from build123d import *

# Parameters (mm, degrees)
SKETCH_1_W          = 30.50790567
SKETCH_1_H          = 76
SKETCH_1_R          = 1.716069694
SKETCH_1_W_2        = 11.5
SKETCH_1_H_2        = 11.5
SKETCH_1_W_3        = 24.50790567
SKETCH_1_H_3        = 19
EXTRUDE_1_DEPTH     = 3.3
SKETCH_2_W          = 30.50790567
SKETCH_2_H          = 6
EXTRUDE_2_DEPTH     = 1
EXTRUDE_3_DEPTH     = 3.3
CUT_EXTRUDE_1_DEPTH = 3.3
SKETCH_8_W          = 30.50790567
SKETCH_8_H          = 29
EXTRUDE_5_DEPTH     = 3.3
CUT_EXTRUDE_3_DEPTH = 3.3
SKETCH_12_W         = 4.466233575
SKETCH_12_H         = 76.29690536
SKETCH_12_W_2       = 3.912291759
SKETCH_12_H_2       = 55.852177881
CUT_EXTRUDE_6_DEPTH = 11.3


with BuildPart() as part:
    # 草圖1 → 填料-伸長1 (new body)
    with BuildSketch(Plane.XY):
        with Locations((0, -4.833822083)):
            Rectangle(SKETCH_1_W, SKETCH_1_H)
        with Locations((-8.65, 10.166177917)):
            Circle(SKETCH_1_R, mode=Mode.SUBTRACT)
        with Locations((-0.03771926, 22.181861337)):
            Rectangle(SKETCH_1_W_2, SKETCH_1_H_2, mode=Mode.SUBTRACT)
        with Locations((8.65, 10.166177917)):
            Circle(SKETCH_1_R, mode=Mode.SUBTRACT)
        with Locations((0, -30.333822083)):
            Rectangle(SKETCH_1_W_3, SKETCH_1_H_3, mode=Mode.SUBTRACT)
    extrude(amount=EXTRUDE_1_DEPTH)

    # 草圖2 → 填料-伸長2 (add)
    with BuildSketch(Plane.XY.offset(3.3)):
        with Locations((0, 1.166177917)):
            Rectangle(SKETCH_2_W, SKETCH_2_H)
        with Locations((0, -10.833822083)):
            Rectangle(SKETCH_2_W, SKETCH_2_H)
    extrude(amount=EXTRUDE_2_DEPTH)

    # 草圖3 → 填料-伸長3 (add)
    with BuildSketch(Plane.XY):
        Polygon((15.253952835, -42.833822083), (-15.253952835, -18.474060109), (15.253952835, -18.474060109), align=None)
    extrude(amount=EXTRUDE_3_DEPTH)

    # 草圖4 → 除料-伸長1 (cut)
    with BuildSketch(Plane.XY.offset(3.3)):
        Polygon((15.253952835, -42.833822083), (-15.253952835, -18.806748841), (-15.253952835, -42.833822083), align=None)
    extrude(amount=-CUT_EXTRUDE_1_DEPTH, mode=Mode.SUBTRACT)

    # 草圖8 → 填料-伸長5 (add)
    with BuildSketch(Plane.XY.offset(3.3)):
        with Locations((0, -28.333822083)):
            Rectangle(SKETCH_8_W, SKETCH_8_H)
    extrude(amount=-EXTRUDE_5_DEPTH)

    # 草圖9 → 除料-伸長3 (cut)
    with BuildSketch(Plane.XY.offset(3.3)):
        Polygon((-15.253952835, -42.833822083), (15.253952835, -18.833822083), (15.253952835, -42.833822083), align=None)
    extrude(amount=-CUT_EXTRUDE_3_DEPTH, mode=Mode.SUBTRACT)

    # 草圖12 → 除料-伸長6 (cut)
    with BuildSketch(Plane.XY.offset(4.3)):
        with Locations((-13.020836048, -4.982274763)):
            Rectangle(SKETCH_12_W, SKETCH_12_H)
        with Locations((14.66842662, 5.240088976)):
            Rectangle(SKETCH_12_W_2, SKETCH_12_H_2)
    extrude(amount=-CUT_EXTRUDE_6_DEPTH, mode=Mode.SUBTRACT)


solid = part.part
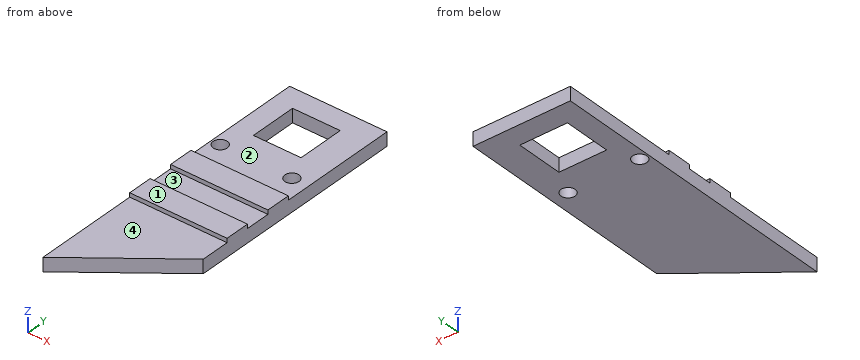
Geometry: final body of the model. Coordinates: model frame, mm. Face numbers are marked on the shaded views. A direction names the side the tool comes from. Coordinates: 2 decimals unless noted, no trailing zeros. Order: outer loops, then holes, each group sorted by start corner. A loop starts at its lowest first (then second) coordinate and runs counter-clockwise, first axis right, second up. Notation, with made-up numbers: M -13.75,58.25 L 1.25,58.25 A19 cw 1.25,64.25 Z; hole C 45.5,55 d6. An arc over 180 degrees is marked long. One line per question, with ' | ' between items. Start each with the question number.
Item 1: Cut plane B-B, the plane x = 8.65. Return the cut outline in (y, z), then the cut area to 3 significant figures.
Item 2: Cut plane C-C, the plane y = 9.5. Return the cut outline in (x, z), then the cut area to 3 significant figures.
Item 3: Set-up query: the marked faces 1, 2, 3 and 4. Return all of +Z, -Z, +X, -X, +Y, -Y with unobstructed straight access to the full face (end or side cutting, diameter ignored); none if empty.
Item 4: Cut plane A-A, the plane y = 26.5. Return the cut outline in (x, z).
Item 5: Pin query (flat end, axial travel): pin 1 Ø1.5 at (y, z) = (-27, 3.5) entering from +X; pin 2 Ø1 at (x, z) = (-1.5, 1.5) entering from -Y; pin 3 Ø1 at (x, y) = (-6.5, 13) entering from -Z; pin 4 Ø1.1 at (x, z) = (0, 4) entering from +Y. Return the tip coordinate at first contact, or that it passes through.
Item 6: Cut plane D-D, the plane z = 0.75. Return the cut outline in (x, y), then the cut area to 3 significant figures.
Item 7: Ray query, probe 1 along X at (y, z) = (20, 0.85); probe 2 along Z at (x, y) = (-8, -6); probe 3 along Y at (x, z) = (9.25, 3.9). Return the intervals inside material, ascending. Write a range as [from, to].
A:
1) outline: M -24.03,0 L 8.45,0 L 8.45,3.3 L 4.17,3.3 L 4.17,4.3 L -1.83,4.3 L -1.83,3.3 L -7.83,3.3 L -7.83,4.3 L -13.83,4.3 L -13.83,3.3 L -24.03,3.3 Z; M 11.88,0 L 33.17,0 L 33.17,3.3 L 11.88,3.3 Z | area: 189 mm2
2) outline: M -10.79,0 L -10.23,0 L -10.23,3.3 L -10.79,3.3 Z; M -7.07,0 L 7.07,0 L 7.07,3.3 L -7.07,3.3 Z; M 10.23,0 L 12.71,0 L 12.71,3.3 L 10.23,3.3 Z | area: 56.7 mm2
3) face 1: +Z, +X, -X, +Y, -Y | face 2: +Z, +X, -X, +Y | face 3: +Z, +X, -X | face 4: +Z, +X, -X, -Y
4) outline: M -10.79,0 L -5.79,0 L -5.79,3.3 L -10.79,3.3 Z; M 5.71,0 L 12.71,0 L 12.71,3.3 L 5.71,3.3 Z
5) pin 1: stops at x = 5.79 | pin 2: stops at y = -32.41 | pin 3: stops at z = 0 | pin 4: stops at y = 4.17
6) outline: M -10.79,-39.32 L 12.71,-20.83 L 12.71,33.17 L -10.79,33.17 Z; hole C -8.65,10.17 d3.43; hole M -5.79,16.43 L 5.71,16.43 L 5.71,27.93 L -5.79,27.93 Z; hole C 8.65,10.17 d3.43 | area: 1,340 mm2
7) probe 1: x = [-10.79, -5.79], [5.71, 12.71] | probe 2: z = [0, 3.3] | probe 3: y = [-13.83, -7.83], [-1.83, 4.17]
